Model file for the job. Use its own axes, mm. Coordinates: 2 decimals unless noted, no trailing zeros. Order: outer loops, then holes, each group sorted by start corner. A loop starts at its lowest first (then second) coordinate and runs counter-clockwise, first axis right, second up. Notation, with made-up numbers: (-9, 13) - (33, 13) arc R17 ccw to (33, 42) - close; hole circle Ø10 at (-33, -8.5). An arc over 180 degrees is marked (long way). Put each result on its own line as item: value. Start each with the question number.
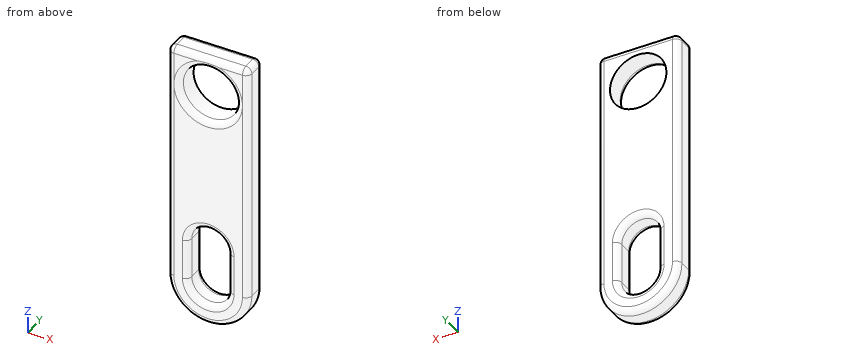
```python
from build123d import *

# Parameters (mm, degrees)
SKETCH1_R           = 3.5
BOSS_EXTRUDE1_DEPTH = 3
FILLET1_R           = 0.75


with BuildPart() as part:
    # Sketch1 → Boss-Extrude1 (new body)
    with BuildSketch(Plane(origin=(0, 0, 0), x_dir=(1, 0, 0), z_dir=(0, 1, 0))):
        with BuildLine():
            Line((-5, -37.44915748), (5, -37.44915748))
            Line((5, -37.44915748), (5, -7.44915748))
            ThreePointArc((5, -7.44915748), (0, -2.44915748), (-5, -7.44915748))
            Line((-5, -7.44915748), (-5, -37.44915748))
        make_face()
        with Locations(Location((0, -32.64915748, 0), (0, 0, 270))):
            Circle(SKETCH1_R, mode=Mode.SUBTRACT)
        with BuildLine():
            Line((2.45, -7.44915748), (2.45, -12.44915748))
            ThreePointArc((2.45, -12.44915748), (0, -14.89915748), (-2.45, -12.44915748))
            Line((-2.45, -12.44915748), (-2.45, -7.44915748))
            ThreePointArc((-2.45, -7.44915748), (0, -4.99915748), (2.45, -7.44915748))
        make_face(mode=Mode.SUBTRACT)
    extrude(amount=BOSS_EXTRUDE1_DEPTH)

    # Fillet1
    # the kernel refuses this fillet: 0.75 mm, written as the material it takes off along each edge
    with BuildSketch(Plane(origin=(-4.25, 2.25, 36.69915748), x_dir=(0, 0, 1), z_dir=(-1, 0, 0))) as fillet1_piece_1_section:
        Polygon((0, 0), (FILLET1_R, 0), (FILLET1_R, FILLET1_R), (0, FILLET1_R), align=None)
    fillet1_piece_1 = extrude(amount=FILLET1_R, mode=Mode.PRIVATE)
    fillet1_piece_1 = fillet1_piece_1 - Plane(origin=(-4.25, 2.25, 36.69915748), x_dir=(0, -0.7071067811865475, -0.7071067811865475), z_dir=(-1, 0, 0)) * Sphere(FILLET1_R, mode=Mode.PRIVATE)
    add(fillet1_piece_1, mode=Mode.SUBTRACT)
    with BuildSketch(Plane(origin=(4.25, 2.25, 36.69915748), x_dir=(0, 1, 0), z_dir=(0, 0, 1))) as fillet1_piece_2_section:
        Polygon((0, 0), (FILLET1_R, 0), (FILLET1_R, -FILLET1_R), (0, -FILLET1_R), align=None)
    fillet1_piece_2 = extrude(amount=FILLET1_R, mode=Mode.PRIVATE)
    fillet1_piece_2 = fillet1_piece_2 - Plane(origin=(4.25, 2.25, 36.69915748), x_dir=(-0.7071067811865475, -0.7071067811865475, 0), z_dir=(0, 0, 1)) * Sphere(FILLET1_R, mode=Mode.PRIVATE)
    add(fillet1_piece_2, mode=Mode.SUBTRACT)
    with BuildSketch(Plane(origin=(-4.25, 0.75, 36.69915748), x_dir=(0, 0, 1), z_dir=(-1, 0, 0))) as fillet1_piece_3_section:
        Polygon((0, 0), (FILLET1_R, 0), (FILLET1_R, -FILLET1_R), (0, -FILLET1_R), align=None)
    fillet1_piece_3 = extrude(amount=FILLET1_R, mode=Mode.PRIVATE)
    fillet1_piece_3 = fillet1_piece_3 - Plane(origin=(-4.25, 0.75, 36.69915748), x_dir=(0, 0.7071067811865475, -0.7071067811865475), z_dir=(-1, 0, 0)) * Sphere(FILLET1_R, mode=Mode.PRIVATE)
    add(fillet1_piece_3, mode=Mode.SUBTRACT)
    with BuildSketch(Plane(origin=(4.25, 0.75, 36.69915748), x_dir=(1, 0, 0), z_dir=(0, 0, 1))) as fillet1_piece_4_section:
        Polygon((0, 0), (FILLET1_R, 0), (FILLET1_R, -FILLET1_R), (0, -FILLET1_R), align=None)
    fillet1_piece_4 = extrude(amount=FILLET1_R, mode=Mode.PRIVATE)
    fillet1_piece_4 = fillet1_piece_4 - Plane(origin=(4.25, 0.75, 36.69915748), x_dir=(-0.7071067811865475, 0.7071067811865475, 0), z_dir=(0, 0, 1)) * Sphere(FILLET1_R, mode=Mode.PRIVATE)
    add(fillet1_piece_4, mode=Mode.SUBTRACT)
    with BuildSketch(Plane(origin=(-5, 3, 7.44915748), x_dir=(0, -1, 0), z_dir=(0, 0, 1)), Plane(origin=(5, 3, 36.69915748), x_dir=(0, -1, 0), z_dir=(0, 0, -1))) as fillet1_piece_5:
        with BuildLine():
            CenterArc((FILLET1_R, FILLET1_R), FILLET1_R, 180, 90)
            Line((0, FILLET1_R), (0, 0))
            Line((0, 0), (FILLET1_R, 0))
        make_face()
    extrude(amount=29.25, mode=Mode.SUBTRACT)
    with BuildSketch(Plane(origin=(0, 0, 7.44915748), x_dir=(-1, 0, 0), z_dir=(0, 0, 1))) as fillet1_piece_6:
        with BuildLine():
            CenterArc((2.45 + FILLET1_R, -FILLET1_R), FILLET1_R, 90, 90)
            Line((2.45 + FILLET1_R, 0), (2.45, 0))
            Line((2.45, 0), (2.45, -FILLET1_R))
        make_face()
    revolve(axis=Axis((0, 0, 7.44915748), (0, -1, 0)), revolution_arc=180, mode=Mode.SUBTRACT)
    with BuildSketch(Plane(origin=(-2.45, 0, 12.44915748), x_dir=(0, 1, 0), z_dir=(0, 0, -1)), Plane(origin=(2.45, 0, 7.44915748), x_dir=(0, 1, 0), z_dir=(0, 0, 1))) as fillet1_piece_7:
        with BuildLine():
            CenterArc((FILLET1_R, -FILLET1_R), FILLET1_R, 90, 90)
            Line((0, -FILLET1_R), (0, 0))
            Line((0, 0), (FILLET1_R, 0))
        make_face()
    extrude(amount=5, mode=Mode.SUBTRACT)
    with BuildSketch(Plane(origin=(0, 0, 12.44915748), x_dir=(1, 0, 0), z_dir=(0, 0, -1))) as fillet1_piece_8:
        with BuildLine():
            CenterArc((2.45 + FILLET1_R, -FILLET1_R), FILLET1_R, 90, 90)
            Line((2.45 + FILLET1_R, 0), (2.45, 0))
            Line((2.45, 0), (2.45, -FILLET1_R))
        make_face()
    revolve(axis=Axis((0, 0, 12.44915748), (0, -1, 0)), revolution_arc=180, mode=Mode.SUBTRACT)
    with BuildSketch(Plane(origin=(0, 3, 7.44915748), x_dir=(-1, 0, 0), z_dir=(0, 0, 1))) as fillet1_piece_9:
        with BuildLine():
            CenterArc((2.45 + FILLET1_R, FILLET1_R), FILLET1_R, 180, 90)
            Line((2.45 + FILLET1_R, 0), (2.45, 0))
            Line((2.45, 0), (2.45, FILLET1_R))
        make_face()
    revolve(axis=Axis((0, 3, 7.44915748), (0, -1, 0)), revolution_arc=180, mode=Mode.SUBTRACT)
    with BuildSketch(Plane(origin=(-4.25, 3, 37.44915748), x_dir=(0, -1, 0), z_dir=(1, 0, 0))) as fillet1_piece_10:
        with BuildLine():
            CenterArc((FILLET1_R, FILLET1_R), FILLET1_R, 180, 90)
            Line((0, FILLET1_R), (0, 0))
            Line((0, 0), (FILLET1_R, 0))
        make_face()
    extrude(amount=8.5, mode=Mode.SUBTRACT)
    with BuildSketch(Plane(origin=(-2.45, 3, 12.44915748), x_dir=(0, -1, 0), z_dir=(0, 0, -1)), Plane(origin=(2.45, 3, 7.44915748), x_dir=(0, -1, 0), z_dir=(0, 0, 1))) as fillet1_piece_11:
        with BuildLine():
            CenterArc((FILLET1_R, FILLET1_R), FILLET1_R, 180, 90)
            Line((0, FILLET1_R), (0, 0))
            Line((0, 0), (FILLET1_R, 0))
        make_face()
    extrude(amount=5, mode=Mode.SUBTRACT)
    with BuildSketch(Plane(origin=(0, 3, 12.44915748), x_dir=(1, 0, 0), z_dir=(0, 0, -1))) as fillet1_piece_12:
        with BuildLine():
            CenterArc((2.45 + FILLET1_R, FILLET1_R), FILLET1_R, 180, 90)
            Line((2.45 + FILLET1_R, 0), (2.45, 0))
            Line((2.45, 0), (2.45, FILLET1_R))
        make_face()
    revolve(axis=Axis((0, 3, 12.44915748), (0, -1, 0)), revolution_arc=180, mode=Mode.SUBTRACT)
    with BuildSketch(Plane(origin=(0, 0, 32.64915748), x_dir=(0, 0, 1), z_dir=(-1, 0, 0))) as fillet1_piece_13:
        with BuildLine():
            CenterArc((3.5 + FILLET1_R, FILLET1_R), FILLET1_R, 180, 90)
            Line((3.5 + FILLET1_R, 0), (3.5, 0))
            Line((3.5, 0), (3.5, FILLET1_R))
        make_face()
    revolve(axis=Axis((0, 0, 32.64915748), (0, 1, 0)), mode=Mode.SUBTRACT)
    with BuildSketch(Plane(origin=(-4.25, 0, 37.44915748), x_dir=(0, 1, 0), z_dir=(1, 0, 0))) as fillet1_piece_14:
        with BuildLine():
            CenterArc((FILLET1_R, -FILLET1_R), FILLET1_R, 90, 90)
            Line((0, -FILLET1_R), (0, 0))
            Line((0, 0), (FILLET1_R, 0))
        make_face()
    extrude(amount=8.5, mode=Mode.SUBTRACT)
    with BuildSketch(Plane(origin=(-5, 0, 7.44915748), x_dir=(0, 1, 0), z_dir=(0, 0, 1)), Plane(origin=(5, 0, 36.69915748), x_dir=(0, 1, 0), z_dir=(0, 0, -1))) as fillet1_piece_15:
        with BuildLine():
            CenterArc((FILLET1_R, -FILLET1_R), FILLET1_R, 90, 90)
            Line((0, -FILLET1_R), (0, 0))
            Line((0, 0), (FILLET1_R, 0))
        make_face()
    extrude(amount=29.25, mode=Mode.SUBTRACT)
    with BuildSketch(Plane(origin=(0, 0, 7.44915748), x_dir=(1, 0, 0), z_dir=(0, 0, 1))) as fillet1_piece_16:
        with BuildLine():
            CenterArc((5 - FILLET1_R, FILLET1_R), FILLET1_R, 270, 90)
            Line((5 - FILLET1_R, 0), (5, 0))
            Line((5, 0), (5, FILLET1_R))
        make_face()
    revolve(axis=Axis((0, 0, 7.44915748), (0, 1, 0)), revolution_arc=180, mode=Mode.SUBTRACT)
    with BuildSketch(Plane(origin=(5, 0.75, 37.44915748), x_dir=(-1, 0, 0), z_dir=(0, 1, 0)), Plane(origin=(-5, 0.75, 37.44915748), x_dir=(0, 0, -1), z_dir=(0, 1, 0))) as fillet1_piece_17:
        with BuildLine():
            CenterArc((FILLET1_R, -FILLET1_R), FILLET1_R, 90, 90)
            Line((0, -FILLET1_R), (0, 0))
            Line((0, 0), (FILLET1_R, 0))
        make_face()
    extrude(amount=1.5, mode=Mode.SUBTRACT)
    with BuildSketch(Plane(origin=(0, 3, 7.44915748), x_dir=(1, 0, 0), z_dir=(0, 0, 1))) as fillet1_piece_18:
        with BuildLine():
            CenterArc((5 - FILLET1_R, -FILLET1_R), FILLET1_R, 0, 90)
            Line((5 - FILLET1_R, 0), (5, 0))
            Line((5, 0), (5, -FILLET1_R))
        make_face()
    revolve(axis=Axis((0, 3, 7.44915748), (0, 1, 0)), revolution_arc=180, mode=Mode.SUBTRACT)


solid = part.part
```
Item 1: Slice it at D-D, the plane x = -2. Give the number of separate pieces and of enclosed holes in the cut face, plus the area to 3 significant figures.
Item 2: Slice it at B-B, the plane y = 1.4. Give the cut face in (x, z).
Item 3: Slice it at A-A, the plane z = 18.5. Give the cut face in (x, y).
Item 4: Slice it at C-C, the plane x = 0. Give the cut face in (y, z).
Item 5: Wall check: line 1 along X through (y, z) = (1.9, 32.5); line 2 along Z through (x, y) = (2.25, 2.2); line 3 along Z through (x, y) = (0.75, 2.85). Give the ranges that are in metal, low to high.
Here are the results:
1. separate pieces: 3
1. enclosed holes: 0
1. area: 61.5 mm^2
2. outline: (-5, 7.45) arc R5 ccw to (5, 7.45) - (5, 36.7) arc R0.75 ccw to (4.25, 37.45) - (-4.25, 37.45) arc R0.75 ccw to (-5, 36.7) - close; hole circle Ø7 at (0, 32.65); hole (-2.45, 7.45) arc R2.45 ccw to (2.45, 7.45) - (2.45, 12.45) arc R2.45 ccw to (-2.45, 12.45) - close
3. outline: (-5, 0.75) arc R0.75 ccw to (-4.25, 0) - (4.25, 0) arc R0.75 ccw to (5, 0.75) - (5, 2.25) arc R0.75 ccw to (4.25, 3) - (-4.25, 3) arc R0.75 ccw to (-5, 2.25) - close
4. outline: (0, 3.2) arc R0.75 ccw to (0.75, 2.45) - (2.25, 2.45) arc R0.75 ccw to (3, 3.2) - (3, 4.25) arc R0.75 ccw to (2.25, 5) - (0.75, 5) arc R0.75 ccw to (0, 4.25) - close; (0, 15.65) arc R0.75 ccw to (0.75, 14.9) - (2.25, 14.9) arc R0.75 ccw to (3, 15.65) - (3, 29.15) - (0.75, 29.15) arc R0.75 ccw to (0, 28.4) - close; (0.01, 36.8) arc R0.75 ccw to (0.75, 36.15) - (3, 36.15) - (3, 36.7) arc R0.75 ccw to (2.25, 37.45) - (0.75, 37.45) arc R0.75 ccw to start
5. line 1: x = -5 to -3.5, 3.5 to 5
5. line 2: z = 2.98 to 6.48, 13.42 to 29.97, 35.33 to 37.45
5. line 3: z = 2.81 to 4.8, 15.09 to 29.23, 36.07 to 37.15
